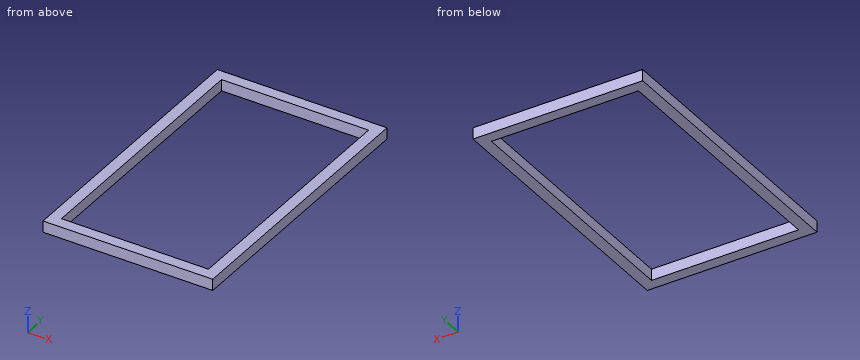
Autodesk Inventor part; units mm, degrees
ref_plane "YZ Plane" through (0, 0, 0) normal (1, 0, 0) x (0, 1, 0)
ref_plane "XZ Plane" through (0, 0, 0) normal (0, 1, 0) x (-1, 0, 0)
ref_plane "XY Plane" through (0, 0, 0) normal (0, 0, 1) x (1, 0, 0)
sketch "Sketch1" plane through (0, 0, 0) normal (0, 0, 1) x (1, 0, 0)
  line L0 (0, 0) -> (190.5, 0)
  line L1 (190.5, 0) -> (190.5, 622.3)
  line L2 (190.5, 622.3) -> (0, 622.3)
  line L3 (0, 0) -> (0, 622.3) construction
  line L4 (0, 0) -> (-190.5, 0)
  line L5 (-190.5, 0) -> (-190.5, 622.3)
  line L6 (-190.5, 622.3) -> (0, 622.3)
  line L7 (-165.1, 25.4) -> (165.1, 25.4)
  line L8 (165.1, 25.4) -> (165.1, 596.9)
  line L9 (165.1, 596.9) -> (-165.1, 596.9)
  line L10 (-165.1, 596.9) -> (-165.1, 25.4)
  dimension "d1" = 622.3
  dimension "d2" = 381
  dimension "d3" = 25.4
  dimension "d4" = 25.4
  dimension "d5" = 25.4
  dimension "d6" = 25.4
extrude "Extrusion1" add sketch "Sketch1" along normal mid plane 25.4
properties part number "primativeBaseForShortRobot"
Can you work these out from the model? Positions are in its coordinate system, mm. Give positions to 0.01 mm unless a question says otherwise; leave off trailing zeros. Loops run counter-clockwise (first coordinate to the right, second up) from the corner with the lowest first, then second, coordinate; pieces in that order, holes last. Notation, with made-up numbers: M 0.25,46 L 59.25,46 A5 ccw 59.25,52 Z; hole C -1,80 d5. An arc over 180 degrees is marked long. One line per question, with ' | ' between items. Start each with the question number.
Q1. If we section it at B-B (x = -110): Please give me the cut outline in (y, z), plus the area to 3 significant figures.
Q2. If I drill on line 1 (Y direction, x = -30, z = 6.75); line 2 (X direction, y = 160.5, z = 1.5), over which ranges is the centre line in solid material (lowest first)? Write a range as from..to.
Q3. If we section it at C-C (z = 0): Please give me the cut outline in (x, y), plus the area to 3 significant figures.
Q4. If we section it at A-A (y = 283): Please give me the cut outline in (x, z), plus the area to 3 significant figures.
Computed:
1) outline: M 0,-12.7 L 25.4,-12.7 L 25.4,12.7 L 0,12.7 Z; M 596.9,-12.7 L 622.3,-12.7 L 622.3,12.7 L 596.9,12.7 Z | area: 1,290 mm²
2) line 1: y = 0..25.4, 596.9..622.3 | line 2: x = -190.5..-165.1, 165.1..190.5
3) outline: M -190.5,0 L 190.5,0 L 190.5,622.3 L -190.5,622.3 Z; hole M -165.1,25.4 L 165.1,25.4 L 165.1,596.9 L -165.1,596.9 Z | area: 48,400 mm²
4) outline: M -190.5,-12.7 L -165.1,-12.7 L -165.1,12.7 L -190.5,12.7 Z; M 165.1,-12.7 L 190.5,-12.7 L 190.5,12.7 L 165.1,12.7 Z | area: 1,290 mm²
